Could you check a few things on this model? Use its own coordinates, in mm. Face numbers are marked on the shaded views. A direction names the side the tool comes from. Round coordinates to 2 decimals unless told otherwise and drop trailing zeros. Loops run counter-clockwise (first coordinate to the right, second up) from the corner with the lowest first, then second, coordinate; pieces in that order, holes last. Notation, with made-up numbers: (43.5, -26.75) - (90.5, -26.75) arc R28 ccw to (90.5, 9.25) - close; hole circle Ø7 at (4, 53.25). An arc over 180 degrees is marked (long way). Use one line per item in the form item = value.
```python
from build123d import *


with BuildPart() as part:
    # Sketch → Revolution (revolve)
    with BuildSketch(Plane.XZ):
        Polygon((14.55, 0), (11.55, 0), (11.55, -2.3), (13.275, -2.3), (13.275, -3.7), (10.3, -6.675), (10.3, 2.5), (7.75, 2.5), (7.75, 4.5), (5.75, 4.5), (5.75, 6.5), (2.75, 6.5), (2.75, 8.5), (0, 8.5), (0, 10.5), (4.75, 10.5), (4.75, 8.5), (7.75, 8.5), (7.75, 6.5), (9.75, 6.5), (9.75, 4.5), (11.9, 4.5), (11.9, 2.5), (14.55, 2.5), align=None)
    revolve(axis=Axis((0, 0, 0), (0, 0, 1)))


solid = part.part
```
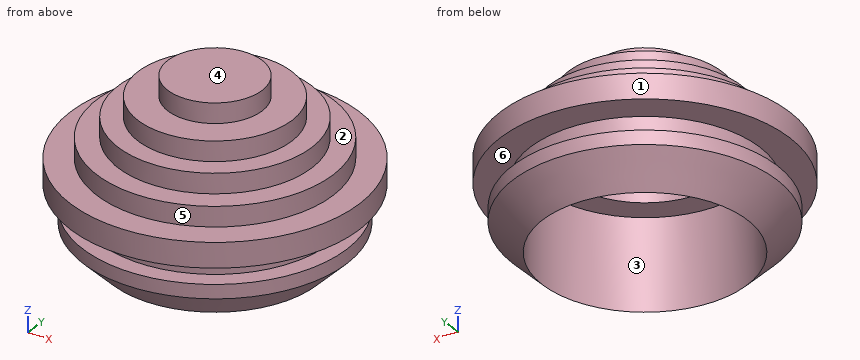
1. We'd pull the mould along Y, two halves only. Please class the marked faces 1, 2 and 3: +Y half, -Y half, draft (parallel to the pull), parting line (faces both ways), or undercut.
Solution:
face_1 = parting line
face_2 = draft
face_3 = undercut
2. On a 3-axis mill with a long thin cutter (end or side, diameter ignored), from which of +Z, -Z, +X, -X, +Y, -Y can I reach the whole of each face in a straight line? I mean the marked faces 4, 5 and 6. Say none if no direction works.
Solution:
face_4 = +Z, +X, -X, +Y, -Y
face_5 = +Z
face_6 = none
3. For P1, Ø13, axis at x = 0, y = 0, coming from the -Z side; P2, Ø3.5, axis at x = 0, y = 0, coming from the -Z side; P3, Ø1.5, axis at x = 8, y = -10.5, coming from the -Z side, each with a flat end and sliding along its axis, tell me the tip position at first contact or that it passes through.
Solution:
P1 = 4.5
P2 = 8.5
P3 = -4.52
4. Please list where these lines run through material, in increasing order: line 1 along Y through (x, z) = (0, 7.75); line 2 along Y through (x, z) = (0, 3.4); line 3 along Z through (x, y) = (-12, -0.75).
Solution:
line_1 = -7.75 to -2.75, 2.75 to 7.75
line_2 = -11.9 to -7.75, 7.75 to 11.9
line_3 = -4.95 to -2.3, 0 to 2.5
5. If we section it at A-A, the plane z = 6: Write out the boundary of the cut face in (x, y), plus the area to 3 significant figures.
Solution:
outline = circle Ø19.5 at (0, 0); hole circle Ø11.5 at (0, 0)
area = 195 mm^2
